Part model, mm, in its own coordinate system. Face numbers are marked on the shaded views. A direction names the side the tool comes from. Round coordinates to 2 decimals unless told otherwise and drop trailing zeros. Write each loop counter-clockwise with the first axis right and the second up, starting at its lowest first coordinate (ties: lowest second). Pieces come first, ordered by that corner, then holes. Notation, with made-up numbers: M 65,55 L 79,55 A14 ccw 79,76 Z; hole C 19,-35.5 d4. An arc over 180 degrees is marked long. Use a Markdown table: item, result. Add a question column.
1) Slice it at A-A on z = 15.5. Write the cut outline in (x, y), plus the area to 3 significant figures.
2) Drop flat-ended pins along their axis: P1, Ø12, axis at x = -56.5, z = 22, coming from the -Y side; P2, Ø1, axis at x = -25.5, z = 17, coming from the +Y side; P3, Ø6, axis at y = -20.5, z = 10, coming from the +X side. Give the stop position or say it passes through.
3) Which spindle directions (+Z, -Z, +X, -X, +Y, -Y) get a long thin tool onto all of the face, cutting with end or side? Do the marked faces 1 and 2. Say none if no direction does.
4) Wall check: probe 1 along Y at (x, z) = (-47, 21.5); probe 2 along X at (y, z) = (-39, 47.5); probe 3 along X at (y, z) = (-36, 28.5). Give the ranges that are in metal, low to high.
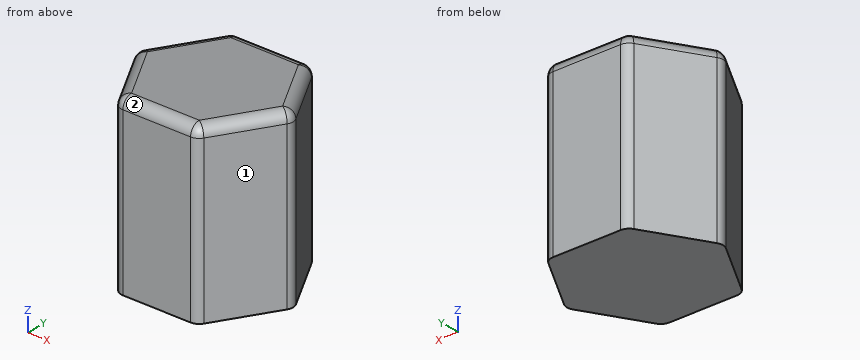
```python
from build123d import *

# Parameters (mm, degrees)
F1_DEPTH = 50
F2_R     = 3


with BuildPart() as f1:
    # F0 (on Top) → F1 (new body)
    with BuildSketch(Plane.XY):
        Polygon((-15.243491, -32.599138), (-26.965457, -12.548407), (-50.190882, -12.674562), (-61.694341, -32.851448), (-49.972375, -52.902179), (-26.74695, -52.776024), align=None)
    extrude(amount=F1_DEPTH)

    # F2
    f2_edges = [f1.edges().sort_by_distance(p)[0] for p in [
        (-38.578169, -12.611485, 50),
        (-55.942612, -22.763005, 50),
        (-55.833358, -42.876814, 50),
        (-21.104474, -22.573773, 50),
        (-38.359663, -52.839102, 50),
        (-20.99522, -42.687581, 50),
        (-50.190882, -12.674562, 25),
        (-61.694341, -32.851448, 25),
        (-26.965457, -12.548407, 25),
        (-15.243491, -32.599138, 25),
        (-26.74695, -52.776024, 25),
        (-49.972375, -52.902179, 25),
    ]]
    fillet(f2_edges, radius=F2_R)


solid = f1.part
```
Entries:
| question | item | result |
|---|---|---|
| 1 | outline | M -60.84,-31.35 A3 ccw -60.82,-34.35 L -50.85,-51.41 A3 ccw -48.24,-52.89 L -28.48,-52.79 A3 ccw -25.89,-51.27 L -16.1,-34.1 A3 ccw -16.12,-31.1 L -26.09,-14.04 A3 ccw -28.7,-12.56 L -48.46,-12.67 A3 ccw -51.05,-14.18 Z |
| 1 | area | 1,400 mm^2 |
| 2 | P1 | stops at y = -51.88 |
| 2 | P2 | stops at y = -14.2 |
| 2 | P3 | stops at x = -20.56 |
| 3 | face 1 | +Z, -Z, +X, -Y |
| 3 | face 2 | +Z, +X, -Y |
| 4 | probe 1 | y = -52.89 to -12.66 |
| 4 | probe 2 | x = -58.05 to -18.94 |
| 4 | probe 3 | x = -59.85 to -17.18 |
